from build123d import *

# Parameters (mm, degrees)
SKETCH1_W           = 85.1
SKETCH1_H           = 56
SKETCH1_R           = 1.5
BOSS_EXTRUDE1_DEPTH = 5
SKETCH3_W           = 12
SKETCH3_H           = 5
BOSS_EXTRUDE2_DEPTH = 5
SKETCH4_W           = 25
SKETCH4_H           = 4
BOSS_EXTRUDE3_DEPTH = 10
SKETCH5_W           = 28
SKETCH5_H           = 3
BOSS_EXTRUDE4_DEPTH = 25


with BuildPart() as part:
    # Sketch1 → Boss-Extrude1 (new body)
    with BuildSketch(Plane(origin=(0, 0, 0), x_dir=(1, 0, 0), z_dir=(0, 1, 0))):
        Rectangle(SKETCH1_W, SKETCH1_H)
        with Locations(Location((-18.95, -24.5, 0), (0, 0, 270))):
            Circle(SKETCH1_R, mode=Mode.SUBTRACT)
        with Locations(Location((39.05, -24.5, 0), (0, 0, 270))):
            Circle(SKETCH1_R, mode=Mode.SUBTRACT)
        with Locations(Location((39.05, 24.5, 0), (0, 0, 270))):
            Circle(SKETCH1_R, mode=Mode.SUBTRACT)
        with Locations(Location((-18.95, 24.5, 0), (0, 0, 270))):
            Circle(SKETCH1_R, mode=Mode.SUBTRACT)
    extrude(amount=BOSS_EXTRUDE1_DEPTH)

    # Sketch3 → Boss-Extrude2 (add)
    with BuildSketch(Plane(origin=(0, 5, 0), x_dir=(1, 0, 0), z_dir=(0, 1, 0))):
        with Locations((-33.55, -26.3)):
            Rectangle(SKETCH3_W, SKETCH3_H)
        with Locations((-8.55, -26.3)):
            Rectangle(SKETCH3_W, SKETCH3_H)
        with Locations((3.45, -26.3)):
            Rectangle(SKETCH3_W, SKETCH3_H)
        with Locations((15.45, -26.3)):
            Rectangle(SKETCH3_W, SKETCH3_H)
    extrude(amount=BOSS_EXTRUDE2_DEPTH)

    # Sketch4 → Boss-Extrude3 (add)
    with BuildSketch(Plane(origin=(0, 5, 0), x_dir=(1, 0, 0), z_dir=(0, 1, 0))):
        with Locations((14.05, 26)):
            Rectangle(SKETCH4_W, SKETCH4_H)
    extrude(amount=BOSS_EXTRUDE3_DEPTH)

    # Sketch5 → Boss-Extrude4 (add)
    with BuildSketch(Plane.XY.offset(-24)):
        with Locations((14, 13.5)):
            Rectangle(SKETCH5_W, SKETCH5_H)
    extrude(amount=BOSS_EXTRUDE4_DEPTH)


solid = part.part
Read the model definition and answer for the solid it produces. Units are mm, in the model's axes. A direction names the side the tool comes from. Give positions to 0.01 mm unless a question says otherwise; leave off trailing zeros. Loops run counter-clockwise (first coordinate to the right, second up) from the corner with the lowest first, then second, coordinate; pieces in that order, holes last. Notation, with made-up numbers: (69, 85.5) -> (127, 85.5) arc R23 cw to (127, 110.5) -> close; hole circle Ø8 at (10.25, 44.25). An arc over 180 degrees is marked (long way). Answer as CSV lines item,"result".
Item 1: Find section C-C on z = -2. Give the vertices of the cut face in (x, y), plus the area to 4 significant figures.
Returned:
outline,"(-42.55, 0) -> (42.55, 0) -> (42.55, 5) -> (-42.55, 5) -> close; (0, 12) -> (28, 12) -> (28, 15) -> (0, 15) -> close"
area,"509.5 mm²"
Item 2: For faces 4 (the face through (14, 8, -24)), 5 (the face through (0, 13, -12)), 6 (the face through (3, 10, 26)), 7 (the face through (14, 12, -12)), 8 (the face through (28, 13, -12)), determine the directions among +Z, -Z, +X, -X, +Y, -Y from which every point of the face is accessible in a straight line to the end or side of a thin tool.
Returned:
face 4,"+X, -X"
face 5,"+Z, -Z, -X, +Y"
face 6,"+Z, +X, -X, +Y"
face 7,"+Z, +X, -X"
face 8,"+Z, -Z, +X, +Y"
Item 3: Find section A-A on x = -18.95. Give the vertices of the cut face in (y, z).
Returned:
outline,"(0, -28) -> (5, -28) -> (5, -26) -> (0, -26) -> close; (0, -23) -> (5, -23) -> (5, 23) -> (0, 23) -> close; (0, 26) -> (5, 26) -> (5, 28) -> (0, 28) -> close"
Item 4: Consider line 1 (X direction, y = 3.8, z = -24.5); line 2 (Y direction, x = 27, z = -3.5); line 3 (Y direction, x = 9.5, z = 6). Determine where each line is inside the solid, lowest interval first. Write a range as [from, to].
Returned:
line 1,"x = [-42.55, -20.45], [-17.45, 37.55], [40.55, 42.55]"
line 2,"y = [0, 5], [12, 15]"
line 3,"y = [0, 5]"
Item 5: Find section D-D on z = 11. Give the vertices of the cut face in (x, y), plus the area to 4 significant figures.
Returned:
outline,"(-42.55, 0) -> (42.55, 0) -> (42.55, 5) -> (-42.55, 5) -> close"
area,"425.5 mm²"
Item 6: Each of these flat-tipped pins is pushed along its axis until it touches: pin 1 (1.2 mm diameter, centred on y = 11, z = -26.5, fed in from -X); pin 2 (1.2 mm diameter, centred on y = 8, z = -27, fed in from +X); pin 3 (0.7 mm diameter, centred on x = 27.5, y = 14, fed in from -Z); pin 4 (2 mm diameter, centred on y = 6.5, z = 18, fed in from +X). Where does it stop, or does it pass through?
Returned:
pin 1,"stops at x = 1.55"
pin 2,"stops at x = 26.55"
pin 3,"stops at z = -24"
pin 4,"passes through"
Item 7: Find section B-B on y = 8. Give the vertices of the cut face in (x, z), plus the area to 3 significant figures.
Returned:
outline,"(-39.55, 23.8) -> (-27.55, 23.8) -> (-27.55, 28.8) -> (-39.55, 28.8) -> close; (-14.55, 23.8) -> (21.45, 23.8) -> (21.45, 28.8) -> (-14.55, 28.8) -> close; (1.55, -28) -> (26.55, -28) -> (26.55, -24) -> (1.55, -24) -> close"
area,"340 mm²"
Item 8: Determine the mould class of faces 1 (the face through (3, 7, 28.8)), 2 (the face through (40.06, 2.46, -25.61)), 3 (the face through (26.55, 10, -26)) for opening direction Z: +Z half, -Z half, draft (parallel to the pull), parting line (faces both ways), or undercut.
Returned:
face 1,"+Z half"
face 2,"undercut"
face 3,"draft"
